Could you check a few things on this model? Use its own coordinates, in mm. A direction names the side the tool comes from. Give positions to 0.01 mm unless a question says otherwise; leave off trailing zeros. Order: outer loops, then holes, each group sorted by start corner. A loop starts at its lowest first (then second) coordinate and runs counter-clockwise, first axis right, second up.
from build123d import *

# Parameters (mm, degrees)
F2_R = 1


with BuildPart() as f1:
    # F0 (on Top) → F1 (revolve)
    with BuildSketch(Plane.XY):
        Polygon((2, 27.4), (2, 0), (3.5, 0), (3.5, 25), (4.5, 25), (4.5, 27.4), align=None)
    revolve(axis=Axis((0, 13.997055, 0), (0, 1, 0)))

    # F2
    f2_edges = [f1.edges().sort_by_distance(p)[0] for p in [
        (-4.5, 27.4, 0),
        (-2, 27.4, 0),
    ]]
    fillet(f2_edges, radius=F2_R)


solid = f1.part
Item 1: For faces 1 (the flat face through (-2, 0, 2)), 2 (the flat face through (0, 25, 4)), which set-ups out of +Z, -Z, +X, -X, +Y, -Y let a thin tool reach every point of the face, with its end or its side?
Findings:
face 1: +Z, -Z, +X, -X, -Y
face 2: -Y
Item 2: We'd pull the mould along Z, two halves only. Please class faces 3 (the cylindrical face through (3.233, 12.675, 1.341)), 4 (the cylindrical face through (0, 13, 2)), 5 (the flat face through (3, 27.4, -1)): +Z half, -Z half, draft (parallel to the pull), parting line (faces both ways), or undercut.
Findings:
face 3: parting line
face 4: undercut
face 5: draft
Item 3: Please list where these lines run through material, in increasing order: line 1 along X through (y, z) = (10.5, 0); line 2 along Y through (x, z) = (-2.75, -1).
Findings:
line 1: x = -3.5 to -2, 2 to 3.5
line 2: y = 0 to 27.4
Item 4: Imagine slicing it at B-B on y = 5. List the corners of the cut face in (x, z) for me, then the cut area to 3 significant figures.
Findings:
outline: circle Ø7 at (0, 0); hole circle Ø4 at (0, 0)
area: 25.9 mm2
Item 5: For pin 1 (3.5 mm diameter, centred on x = 0, z = 0, fed in from -Y); pin 2 (4 mm diameter, centred on x = 1, y = 17, fed in from -Z); pin 3 (5 mm diameter, centred on x = 0, z = 0, fed in from +Y), each with a flat end and sliding along its axis, tell me the tip position at first contact or that it passes through.
Findings:
pin 1: passes through
pin 2: stops at z = -3.5
pin 3: stops at y = 27.27
Item 6: Imagine slicing it at A-A on x = 0. List the corners of the cut face in (y, z) for me.
Findings:
outline: (0, -3.5) - (25, -3.5) - (25, -4.5) - (26.4, -4.5) arc R1 ccw to (27.4, -3.5) - (27.4, -3) arc R1 ccw to (26.4, -2) - (0, -2) - close; (0, 2) - (26.4, 2) arc R1 ccw to (27.4, 3) - (27.4, 3.5) arc R1 ccw to (26.4, 4.5) - (25, 4.5) - (25, 3.5) - (0, 3.5) - close
